Build history of the part. All positions in model axes, mm. A direction names the side the tool comes from. Give positions to 0.01 mm unless a question says otherwise; leave off trailing zeros. Order: outer loops, then holes, each group sorted by start corner. A loop starts at its lowest first (then second) coordinate and runs counter-clockwise, first axis right, second up. Notation, with made-up numbers: (3.25, 52) - (18.25, 52) arc R19 ccw to (18.25, 75) - close; hole circle Ø7 at (14.25, -6). An arc over 180 degrees is marked (long way). Write each question's results on one line, items separated by ' | '. Start each with the question number.
1) Cut at A-A on z = -17. List the corners of the cut face in (x, y), plus the area to 3 significant figures.
2) Cut at C-C on z = -40.5. List the corners of the cut face in (x, y).
3) Two-plate mould, pull along Y, no slides. Class faces 1 (the face through (-9.948, 0.713, -7.527)), 2 (the face through (-11.469, 16, -27)), 3 (the face through (-8.04, 10.77, -47.87)): +Y half, -Y half, draft (parallel to the pull), parting line (faces both ways), or undercut.
4) Drop flat-ended pins along their axis: pin 1 Ø2 at (y, z) = (4, -23.5) entering from -X; pin 2 Ø1.5 at (x, z) = (-4.5, -10) entering from +Y; pin 3 Ø4 at (y, z) = (3.5, -40) entering from +X; pin 4 Ø4.5 at (y, z) = (8.11, -5.6) entering from -X. Give the stop position or say it passes through.
5) Cut at B-B on y = -9. List the corners of the cut face in (x, z), plus the area to 3 significant figures.
6) Cut at D-D on y = 3. List the corners of the cut face in (x, z), plus the area to 3 significant figures.
7) Tool access for faces 4 (the face through (-0.4, 7.49, -26.85)), 5 (the face through (-8.469, 4, -6)), 6 (the face through (-0.4, 7.49, -47.87)), 7 (the face through (33.236, -17.51, -26.85)): list every direction of +Z, -Z, +X, -X, +Y, -Y with a clear straight run to the whole face (end or side of a thin tool).
8) Drill centre lines: line 1 along Z through (x, y) = (-8.5, 3); line 2 along X through (y, z) = (10, -7); line 3 along X through (y, z) = (3, -8). Where is each one in solid material? Low to high. Write a range as from..to.
from build123d import *

# Parameters (mm, degrees)
BOSS_EXTRUDE1_DEPTH        = 10
CUT_EXTRUDE1_DEPTH         = 24.288163202
M3_5_CLEARANCE_HOLE1_D     = 4.04
M3_5_CLEARANCE_HOLE1_DEPTH = 11.976330523
M3_5_CLEARANCE_HOLE2_D     = 4.04
M3_5_CLEARANCE_HOLE2_DEPTH = 3
FILLET1_R                  = 2.5
COMBINE1_START             = -42.798318907
COMBINE1_DEPTH             = 32.198103497
COMBINE1_START_2           = -52.798318907
COMBINE1_2_DEPTH           = 10
COMBINE1_3_DEPTH           = 5.304051749
COMBINE1_START_3           = -15.904267158
COMBINE1_4_DEPTH           = 5.304051748


with BuildPart() as part:
    # Sketch1 → Boss-Extrude1 (new body)
    with BuildSketch(Plane.XY.offset(-0.60021541)):
        Polygon((-11.469163068, -7.348185616), (-11.452492295, -7.348185616), (0.507167456, 8.709585816), (-11.469163068, 17.629431184), align=None)
    extrude(amount=-BOSS_EXTRUDE1_DEPTH)

    # Sketch2 → Cut-Extrude1 (cut, through all)
    with BuildSketch(Plane(origin=(0, 0, -10.60021541), x_dir=(-1, 0, 0), z_dir=(0, 0, -1))):
        with BuildLine():
            Line((8.469163068, -3.342585136), (8.469163068, 10.061084473))
            ThreePointArc((8.469163068, 10.061084473), (8.028129493, 10.776027202), (7.191305305, 10.702685563))
            Line((7.191305305, 10.702685563), (1.284799154, 6.303581729))
            Line((1.284799154, 6.303581729), (8.469163068, -3.342585136))
        make_face()
    extrude(amount=-CUT_EXTRUDE1_DEPTH, mode=Mode.SUBTRACT)

    # M3.5 Clearance Hole1
    with Locations(Plane.ZY.offset(11.469163068)):
        with Locations((-5.60021541, 0.106053799)):
            Hole(M3_5_CLEARANCE_HOLE1_D / 2, depth=M3_5_CLEARANCE_HOLE1_DEPTH)

    # M3.5 Clearance Hole2
    with Locations(Plane.ZY.offset(11.469163068)):
        with Locations((-5.60021541, 8.106053799)):
            Hole(M3_5_CLEARANCE_HOLE2_D / 2, depth=M3_5_CLEARANCE_HOLE2_DEPTH)

    # Fillet1
    fillet1_edges = [part.edges().sort_by_distance(p)[0] for p in [
        (-8.469163068, -3.342585136, -5.60021541),
    ]]
    fillet(fillet1_edges, radius=FILLET1_R)

    # Combine1: read off the stored shape, not the designer's step
    # Combine1 outline → Combine1 (add)
    with BuildSketch(Plane.XY.offset(COMBINE1_START)):
        Polygon((-1.284799143, 6.30358172), (0.507167468, 8.709585807), (-11.469163068, 17.629431184), (-11.469163068, 13.888789159), align=None)
        Polygon((40.70546383, -21.229683728), (34.119044566, -16.324187738), (32.327077956, -18.730191825), (38.913497219, -23.635687815), align=None)
    extrude(amount=COMBINE1_DEPTH)

    # Combine1 2 outline → Combine1 2 (add)
    with BuildSketch(Plane.XY.offset(COMBINE1_START_2)):
        with BuildLine():
            Line((-1.284799143, 6.30358172), (0.507167468, 8.709585807))
            Line((0.507167468, 8.709585807), (-11.469163068, 17.629431184))
            Line((-11.469163068, 17.629431184), (-11.469163068, -7.348185616))
            Line((-11.469163068, -7.348185616), (-11.452492295, -7.348185616))
            Line((-11.452492295, -7.348185616), (-8.964159662, -4.00719787))
            ThreePointArc((-8.964159662, -4.00719787), (-8.596136676, -3.300496292), (-8.469163068, -2.513892362))
            Line((-8.469163068, -2.513892362), (-8.469163068, 10.061084473))
            ThreePointArc((-8.469163068, 10.061084473), (-8.028129494, 10.776027202), (-7.191305305, 10.702685563))
            Line((-7.191305305, 10.702685563), (-1.284799143, 6.30358172))
        make_face()
    extrude(amount=COMBINE1_2_DEPTH)

    # Combine1 3 outline → Combine1 3 (add)
    with BuildSketch(Plane.XY.offset(COMBINE1_START)):
        Polygon((34.119044566, -16.324187738), (0.507167462, 8.709585812), (-1.284799143, 6.30358172), (32.327077956, -18.730191825), align=None)
    extrude(amount=COMBINE1_3_DEPTH)

    # Combine1 4 outline → Combine1 4 (add)
    with BuildSketch(Plane.XY.offset(COMBINE1_START_3)):
        Polygon((34.119044566, -16.324187738), (0.507167462, 8.709585812), (-1.284799143, 6.30358172), (32.327077956, -18.730191825), align=None)
    extrude(amount=COMBINE1_4_DEPTH)

    # Combine1 5: loft between two sections, ruled curve by curve
    combine1_5_from = [
        Edge.make_three_point_arc((36.665398892, -18.220685734, -29.759967158), (35.045917541, -17.014513008, -31.779267158), (36.665398892, -18.220685734, -33.798567158)),
        Edge.make_three_point_arc((36.665398892, -18.220685734, -33.798567158), (38.284880243, -19.426858459, -31.779267158), (36.665398892, -18.220685734, -29.759967158)),
    ]
    combine1_5_to = [
        Edge.make_three_point_arc((34.873432281, -20.626689821, -29.759967158), (33.25395093, -19.420517096, -31.779267158), (34.873432281, -20.626689821, -33.798567158)),
        Edge.make_three_point_arc((34.873432281, -20.626689821, -33.798567158), (36.492913632, -21.832862546, -31.779267158), (34.873432281, -20.626689821, -29.759967158)),
    ]
    combine1_5 = Solid(Shell([*[Face.make_surface_from_curves(combine1_5_from[k], combine1_5_to[k]) for k in range(2)], Face(Wire(combine1_5_from)), Face(Wire(combine1_5_to))]))
    add(combine1_5, mode=Mode.SUBTRACT)

    # Combine1 6: loft between two sections, ruled curve by curve
    combine1_6_from = [
        Edge.make_three_point_arc((36.665398892, -18.220685734, -19.599967158), (35.045917541, -17.014513008, -21.619267158), (36.665398892, -18.220685734, -23.638567158)),
        Edge.make_three_point_arc((36.665398892, -18.220685734, -23.638567158), (38.284880243, -19.426858459, -21.619267158), (36.665398892, -18.220685734, -19.599967158)),
    ]
    combine1_6_to = [
        Edge.make_three_point_arc((34.873432281, -20.626689821, -19.599967158), (33.25395093, -19.420517096, -21.619267158), (34.873432281, -20.626689821, -23.638567158)),
        Edge.make_three_point_arc((34.873432281, -20.626689821, -23.638567158), (36.492913632, -21.832862546, -21.619267158), (34.873432281, -20.626689821, -19.599967158)),
    ]
    combine1_6 = Solid(Shell([*[Face.make_surface_from_curves(combine1_6_from[k], combine1_6_to[k]) for k in range(2)], Face(Wire(combine1_6_from)), Face(Wire(combine1_6_to))]))
    add(combine1_6, mode=Mode.SUBTRACT)

    # Combine1 7: loft between two sections, ruled curve by curve
    combine1_7_from = [
        Edge.make_three_point_arc((-2.039186858, 10.606083803, -29.759967158), (-3.658668209, 11.812256529, -31.779267158), (-2.039186858, 10.606083803, -33.798567158)),
        Edge.make_three_point_arc((-2.039186858, 10.606083803, -33.798567158), (-0.419705507, 9.399911078, -31.779267158), (-2.039186858, 10.606083803, -29.759967158)),
    ]
    combine1_7_to = [
        Edge.make_three_point_arc((-3.831153468, 8.200079716, -29.759967158), (-5.45063482, 9.406252441, -31.779267158), (-3.831153468, 8.200079716, -33.798567158)),
        Edge.make_three_point_arc((-3.831153468, 8.200079716, -33.798567158), (-2.211672117, 6.993906991, -31.779267158), (-3.831153468, 8.200079716, -29.759967158)),
    ]
    combine1_7 = Solid(Shell([*[Face.make_surface_from_curves(combine1_7_from[k], combine1_7_to[k]) for k in range(2)], Face(Wire(combine1_7_from)), Face(Wire(combine1_7_to))]))
    add(combine1_7, mode=Mode.SUBTRACT)

    # Combine1 8: loft between two sections, ruled curve by curve
    combine1_8_from = [
        Edge.make_three_point_arc((-2.039186858, 10.606083803, -19.599967158), (-3.658668209, 11.812256529, -21.619267158), (-2.039186858, 10.606083803, -23.638567158)),
        Edge.make_three_point_arc((-2.039186858, 10.606083803, -23.638567158), (-0.419705507, 9.399911078, -21.619267158), (-2.039186858, 10.606083803, -19.599967158)),
    ]
    combine1_8_to = [
        Edge.make_three_point_arc((-3.831153468, 8.200079716, -19.599967158), (-5.45063482, 9.406252441, -21.619267158), (-3.831153468, 8.200079716, -23.638567158)),
        Edge.make_three_point_arc((-3.831153468, 8.200079716, -23.638567158), (-2.211672117, 6.993906991, -21.619267158), (-3.831153468, 8.200079716, -19.599967158)),
    ]
    combine1_8 = Solid(Shell([*[Face.make_surface_from_curves(combine1_8_from[k], combine1_8_to[k]) for k in range(2)], Face(Wire(combine1_8_from)), Face(Wire(combine1_8_to))]))
    add(combine1_8, mode=Mode.SUBTRACT)

    # Combine1 9: loft between two sections, ruled curve by curve
    combine1_9_from = [
        Edge.make_three_point_arc((-8.466516755, 8.106053799, -45.778318907), (-8.466516755, 10.126053799, -47.798318907), (-8.466516755, 8.106053799, -49.818318907)),
        Edge.make_three_point_arc((-8.466516755, 8.106053799, -49.818318907), (-8.466516755, 6.086053799, -47.798318907), (-8.466516755, 8.106053799, -45.778318907)),
    ]
    combine1_9_to = [
        Edge.make_three_point_arc((-11.469163068, 8.106053799, -45.778318907), (-11.469163068, 10.126053799, -47.798318907), (-11.469163068, 8.106053799, -49.818318907)),
        Edge.make_three_point_arc((-11.469163068, 8.106053799, -49.818318907), (-11.469163068, 6.086053799, -47.798318907), (-11.469163068, 8.106053799, -45.778318907)),
    ]
    combine1_9 = Solid(Shell([*[Face.make_surface_from_curves(combine1_9_from[k], combine1_9_to[k]) for k in range(2)], Face(Wire(combine1_9_from)), Face(Wire(combine1_9_to))]))
    add(combine1_9, mode=Mode.SUBTRACT)

    # Combine1 10: loft between two sections, ruled curve by curve
    combine1_10_from = [
        Edge.make_three_point_arc((-8.469163068, 0.106053799, -45.778318907), (-8.469163068, 2.126053799, -47.798318907), (-8.469163068, 0.106053799, -49.818318907)),
        Edge.make_three_point_arc((-8.469163068, 0.106053799, -49.818318907), (-8.469163068, -1.913946201, -47.798318907), (-8.469163068, 0.106053799, -45.778318907)),
    ]
    combine1_10_to = [
        Edge.make_three_point_arc((-11.469163068, 0.106053799, -45.778318907), (-11.469163068, 2.126053799, -47.798318907), (-11.469163068, 0.106053799, -49.818318907)),
        Edge.make_three_point_arc((-11.469163068, 0.106053799, -49.818318907), (-11.469163068, -1.913946201, -47.798318907), (-11.469163068, 0.106053799, -45.778318907)),
    ]
    combine1_10 = Solid(Shell([*[Face.make_surface_from_curves(combine1_10_from[k], combine1_10_to[k]) for k in range(2)], Face(Wire(combine1_10_from)), Face(Wire(combine1_10_to))]))
    add(combine1_10, mode=Mode.SUBTRACT)


solid = part.part
Results:
1) outline: (-11.47, 13.89) - (-1.28, 6.3) - (0.51, 8.71) - (-11.47, 17.63) - close; (32.33, -18.73) - (38.91, -23.64) - (40.71, -21.23) - (34.12, -16.32) - close | area: 66.1 mm^2
2) outline: (-11.47, 13.89) - (38.91, -23.64) - (40.71, -21.23) - (-11.47, 17.63) - close
3) face 1: undercut | face 2: draft | face 3: -Y half
4) pin 1: through | pin 2: y = 13 | pin 3: x = 10.19 | pin 4: x = -11.47
5) outline: (19.26, -42.8) - (24.29, -42.8) - (24.29, -37.49) - (19.26, -37.49) - close; (19.26, -15.9) - (24.29, -15.9) - (24.29, -10.6) - (19.26, -10.6) - close | area: 53.3 mm^2
6) outline: (-11.47, -52.8) - (-8.47, -52.8) - (-8.47, -42.8) - (-11.47, -42.8) - close; (-11.47, -10.6) - (-8.47, -10.6) - (-8.47, -0.6) - (-11.47, -0.6) - close; (3.15, -42.8) - (8.17, -42.8) - (8.17, -37.49) - (3.15, -37.49) - close; (3.15, -15.9) - (8.17, -15.9) - (8.17, -10.6) - (3.15, -10.6) - close | area: 113 mm^2
7) face 4: +X, -Y | face 5: +Z, -Z, -Y | face 6: -Z, +X, -Y | face 7: -X, +Y
8) line 1: -52.8..-42.8, -10.6..-0.6 | line 2: -11.47..-8.47, -6.25..-1.23 | line 3: -11.47..-8.47
